from build123d import *

# Parameters (mm, degrees)
F1_DEPTH = 4
F3_D     = 19
F4_D     = 12


with BuildPart() as f1:
    # F0 (on Front) → F1 (new body)
    with BuildSketch(Plane.XZ):
        with BuildLine():
            Line((15, -53.838078), (15, 36.104428))
            ThreePointArc((15, 36.104428), (0, 51.162033), (-15, 36.104428))
            Line((-15, 36.104428), (-15, -53.838078))
            ThreePointArc((-15, -53.838078), (0, -68.838078), (15, -53.838078))
        make_face()
    extrude(amount=F1_DEPTH)

    # F3 (through all)
    with Locations(Plane.XZ.offset(4)):
        with Locations((0, 36.161922)):
            Hole(F3_D / 2)

    # F4 (through all)
    with Locations(Plane.XZ.offset(4)):
        with Locations((0, -53.838078)):
            Hole(F4_D / 2)


solid = f1.part
Source: CAD feature listing. Evaluate the final solid. Frame: model axes, mm. Round coordinates to 2 decimals unless told otherwise and drop trailing zeros. Loops run counter-clockwise (first coordinate to the right, second up) from the corner with the lowest first, then second, coordinate; pieces in that order, holes last.
Q1. Section A-A, the plane x = 0. Return loops of the section in (y, z), plus the area to 3 significant figures.
Q2. Ray query, line 1 (Z direction, x = 0, y = -1.8); line 2 (X direction, y = -0.95, z = 36); line 3 (Z direction, x = -1, y = -2.5). Return the intervals inside material, ascending.
Q3. Section C-C, the plane x = -8.5. Return loops of the section in (y, z).
Q4. Mould query, pull axis Z, two halves, no side actions, for faces 1 (the face through (15, -2, -9)), 2 (the face through (-0.33, -1.972, -68.834)), 3 (the face through (2.06, -1.97, 26.89)). Classes: pulls with the +Z half, pulls with the -Z half, needs draft (parallel to the pull), parting line crosses it, or undercut.
Q5. First-contact query: P1, Ø15.5, axis at x = 0, z = -53.84, coming from the -Y side; P2, Ø1.5, axis at x = 7, y = -1, coming from the +Z side. Flat tips, straight axial feed; report the tip coordinate or a pass-through.
Q6. Section D-D, the plane y = -1.7. Return loops of the section in (x, z), plus the area to 3 significant figures.
Q7. Section B-B, the plane z = 42. Return loops of the section in (x, y), plus the area to 3 significant figures.
Solutions:
1. outline: (-4, -68.84) - (0, -68.84) - (0, -59.84) - (-4, -59.84) - close; (-4, -47.84) - (0, -47.84) - (0, 26.66) - (-4, 26.66) - close; (-4, 45.66) - (0, 45.66) - (0, 51.16) - (-4, 51.16) - close
1. area: 356 mm2
2. line 1: z = -68.84 to -59.84, -47.84 to 26.66, 45.66 to 51.16
2. line 2: x = -15 to -9.5, 9.5 to 15
2. line 3: z = -68.8 to -59.75, -47.92 to 26.71, 45.61 to 51.13
3. outline: (-4, -66.2) - (0, -66.2) - (0, 31.92) - (-4, 31.92) - close; (-4, 40.4) - (0, 40.4) - (0, 48.52) - (-4, 48.52) - close
4. face 1: needs draft
4. face 2: pulls with the -Z half
4. face 3: undercut
5. P1: stops at y = -4
5. P2: stops at z = 49.8
6. outline: (-15, -53.84) arc R15 ccw to (15, -53.84) - (15, 36.1) arc R15 ccw (long way) to (-15, 36.1) - close; hole circle Ø19 at (0, 36.16); hole circle Ø12 at (0, -53.84)
6. area: 3,010 mm2
7. outline: (-13.82, -4) - (-7.49, -4) - (-7.49, 0) - (-13.82, 0) - close; (7.49, -4) - (13.82, -4) - (13.82, 0) - (7.49, 0) - close
7. area: 50.6 mm2
